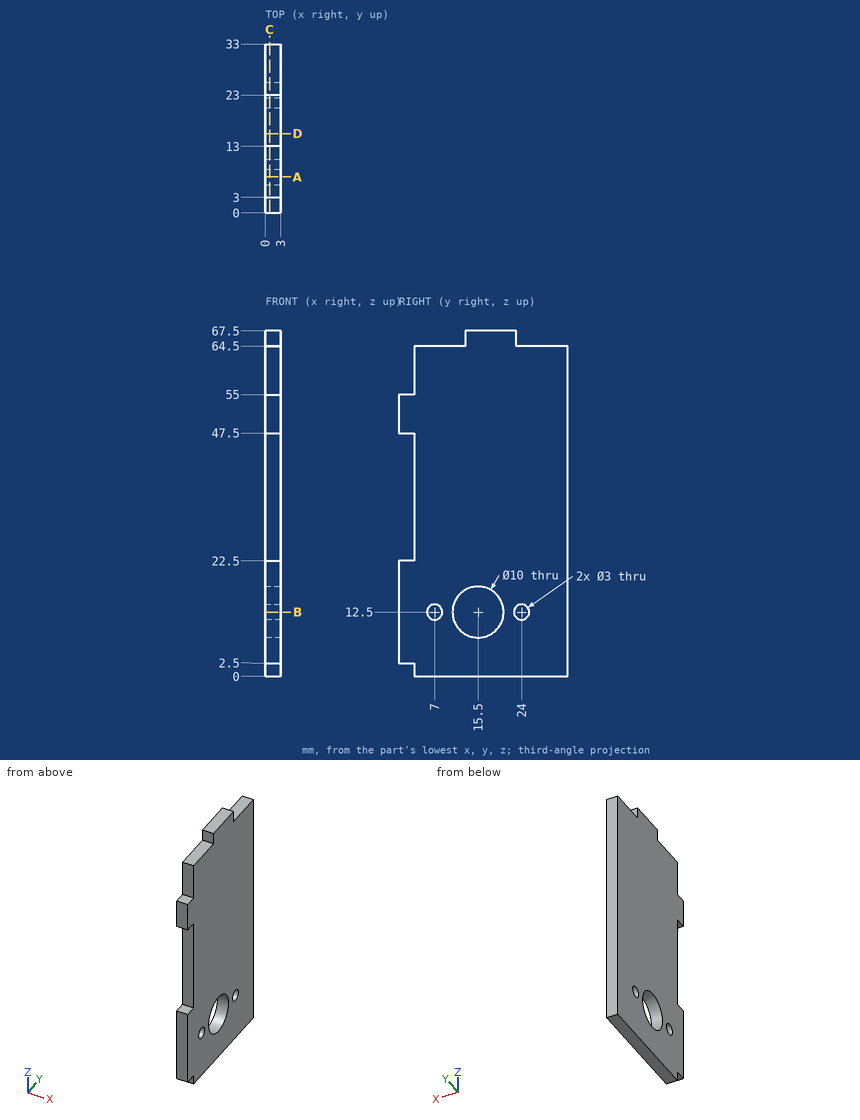
Could you check a few things on this drawing? It's one solid part, dimensions in mm from its lowest x, y, z. Give positions to 0.01 mm unless a question says otherwise; leave off trailing zeros. Loops run counter-clockwise (first coordinate to the right, second up) from the corner with the lowest first, then second, coordinate; pieces in that order, holes last. Notation, with made-up numbers: M 10,8.5 L 63,8.5 A17 ccw 63,24.5 Z; hole C 73.25,82.25 d4. An arc over 180 degrees is marked long. Answer as a JSON object with one key per item and string values.
Q1. Suppose I cut it at D-D, the plane y = 15.5. List the corners of the cut face in (x, z) for me.
Values found:
{"outline": "M 0,0 L 3,0 L 3,7.5 L 0,7.5 Z; M 0,17.5 L 3,17.5 L 3,67.5 L 0,67.5 Z"}
Q2. If I drill on probe 1 along Y at (x, z) = (1.45, 12.5); probe 2 along Z at (x, y) = (1.95, 30.5); probe 3 along Y at (x, z) = (1.4, 23.5), over which ranges is the centre line in solid material (lowest first)? Write a range as [from, to].
Values found:
{"probe 1": "y = [0, 5.5], [8.5, 10.5], [20.5, 22.5], [25.5, 33]", "probe 2": "z = [0, 64.5]", "probe 3": "y = [3, 33]"}
Q3. Suppose I cut it at B-B, the plane z = 12.5. List the corners of the cut face in (x, y) for me.
Values found:
{"outline": "M 0,0 L 3,0 L 3,5.5 L 0,5.5 Z; M 0,8.5 L 3,8.5 L 3,10.5 L 0,10.5 Z; M 0,20.5 L 3,20.5 L 3,22.5 L 0,22.5 Z; M 0,25.5 L 3,25.5 L 3,33 L 0,33 Z"}
Q4. For P1, Ø1.5, axis at x = 2, z = 66, coming from the +Y side; P2, Ø6, axis at y = 20, z = 33, coming from the -X side; P3, Ø1.5, axis at x = 1, y = 8, coming from the +Z side; P4, Ø0.9, axis at x = 2, y = 1.5, coming from the +Z side, each with a flat end and sliding along its axis, tell me the tip position at first contact or that it passes through.
Values found:
{"P1": "stops at y = 23", "P2": "stops at x = 0", "P3": "stops at z = 64.5", "P4": "stops at z = 55"}
Q5. Suppose I cut it at C-C, the plane x = 0.8. List the corners of the cut face in (y, z) for me.
Values found:
{"outline": "M 0,2.5 L 3,2.5 L 3,0 L 33,0 L 33,64.5 L 23,64.5 L 23,67.5 L 13,67.5 L 13,64.5 L 3,64.5 L 3,55 L 0,55 L 0,47.5 L 3,47.5 L 3,22.5 L 0,22.5 Z; hole C 7,12.5 d3; hole C 15.5,12.5 d10; hole C 24,12.5 d3"}
Q6. Suppose I cut it at A-A, the plane y = 7. List the corners of the cut face in (x, z) for me, plus the area to 4 significant figures.
Values found:
{"outline": "M 0,0 L 3,0 L 3,11 L 0,11 Z; M 0,14 L 3,14 L 3,64.5 L 0,64.5 Z", "area": "184.5 mm²"}
